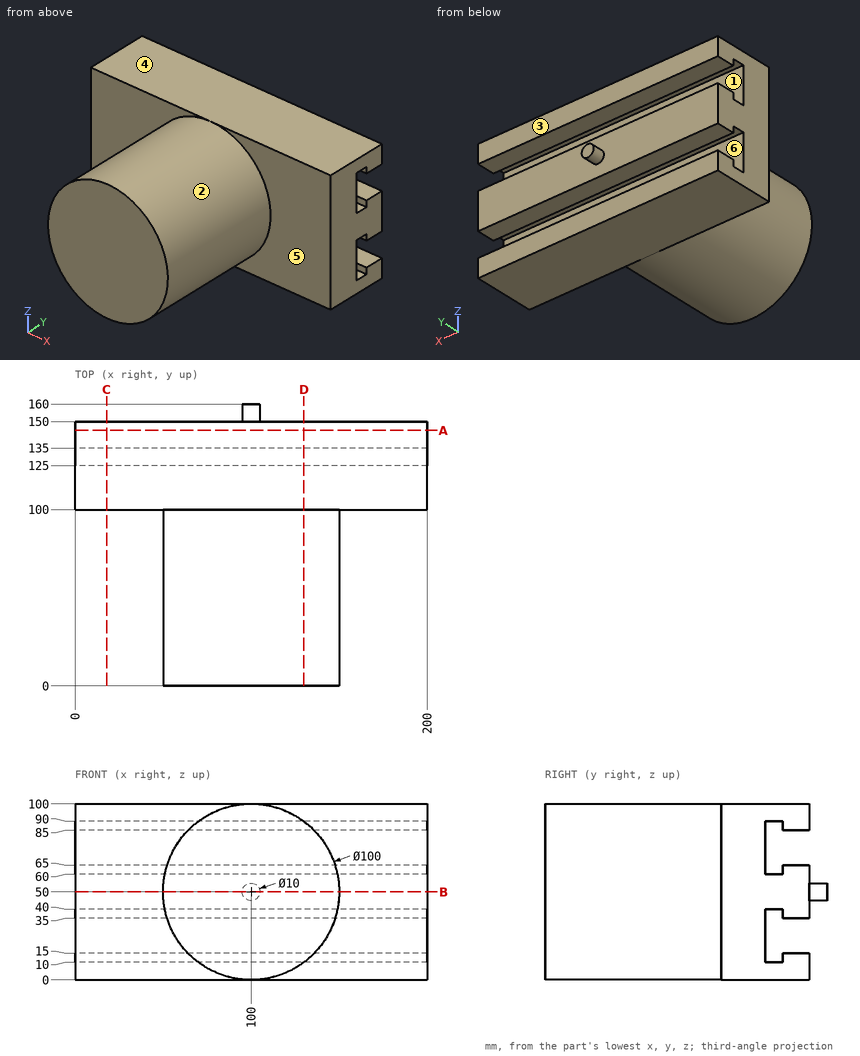
Answer from the drawing. Dimensions are ordinates in mm from the lowest x, y and z of the part. A direction names the side the tool comes from. Give positions to 0.01 mm unless a question says otherwise; leave off trailing zeros. Order: outer loops, then holes, each group sorted by start corner. A loop starts at its lowest first (then second) coordinate and runs counter-clockwise, first axis right, second up. Notation, with made-up numbers: (37, 62) - (63, 62) arc R31 cw to (63, 100) - close; hole circle Ø10 at (-24.75, 22). An arc over 180 degrees is marked (long way). One line per item, written item: value. Start each with the question number.
1) Given pin 1 Ø8 at (x, z) = (165.5, 78) entering from -Y; pin 2 Ø2 at (x, z) = (112.5, 82) entering from +Y; pin 3 Ø9 at (x, z) = (65, 53.5) entering from +Y, each flat-ended and moving along its own axis, determine where each tip first touches the part or whether it passes through.
2) A cutting plane is placed at B-B on z = 50. Give the vertices of the cut face in (x, y).
3) The mould has two halves that part along Z. Classify the marked faces 1, 2 and 3: released by +Z, released by -Z, zero draft, split by the parting line, or undercut.
4) A cutting plane is placed at D-D on x = 130. Give the vertices of the cut face in (y, z), then the cut area to 3 significant figures.
5) Find the intervals of material crossed by L1, parallel to Z at x = 39, y = 148.5; L2, parallel to Z at x = 28, y = 129; L3, parallel to Y at x = 44.5, z = 62, in increasing order.
6) A cutting plane is placed at C-C on x = 18. Give the vertices of the cut face in (y, z), then the cut area to 3 significant figures.
7) A cutting plane is placed at A-A on y = 145. Give the vertices of the cut face in (x, z), then the cut area to 3 significant figures.
8) A tool of negligible diameter and unlimited length cuts with its end or side. For the marked faces 4, 5 and 6, from which of +Z, -Z, +X, -X, +Y, -Y can it reach the whole face along a straight path? Write none if from no direction.
Answer sheet:
1. pin 1: stops at y = 100
1. pin 2: stops at y = 125
1. pin 3: stops at y = 150
2. outline: (0, 100) - (50, 100) - (50, 0) - (150, 0) - (150, 100) - (200, 100) - (200, 150) - (105, 150) - (105, 160) - (95, 160) - (95, 150) - (0, 150) - close
3. face 1: undercut
3. face 2: split by the parting line
3. face 3: zero draft
4. outline: (0, 10) - (100, 10) - (100, 0) - (150, 0) - (150, 15) - (135, 15) - (135, 10) - (125, 10) - (125, 40) - (135, 40) - (135, 35) - (150, 35) - (150, 65) - (135, 65) - (135, 60) - (125, 60) - (125, 90) - (135, 90) - (135, 85) - (150, 85) - (150, 100) - (100, 100) - (100, 90) - (0, 90) - close
4. area: 11,800 mm2
5. L1: z = 0 to 15, 35 to 65, 85 to 100
5. L2: z = 0 to 10, 40 to 60, 90 to 100
5. L3: y = 100 to 125, 135 to 150
6. outline: (100, 0) - (150, 0) - (150, 15) - (135, 15) - (135, 10) - (125, 10) - (125, 40) - (135, 40) - (135, 35) - (150, 35) - (150, 65) - (135, 65) - (135, 60) - (125, 60) - (125, 90) - (135, 90) - (135, 85) - (150, 85) - (150, 100) - (100, 100) - close
6. area: 3,800 mm2
7. outline: (0, 0) - (200, 0) - (200, 15) - (0, 15) - close; (0, 35) - (200, 35) - (200, 65) - (0, 65) - close; (0, 85) - (200, 85) - (200, 100) - (0, 100) - close
7. area: 12,000 mm2
8. face 4: +Z, +X, -X, +Y, -Y
8. face 5: +X, -Y
8. face 6: +X, -X
